Can you work these out from the model? Positions are in its coordinate system, mm. A direction names the side the tool comes from. Round coordinates to 2 decimals unless told otherwise and drop trailing zeros. Loops run counter-clockwise (first coordinate to the right, second up) from the corner with the lowest first, then second, coordinate; pieces in that order, holes last.
```python
from build123d import *

# Parameters (mm, degrees)
ESQUISSE1_W             = 30
ESQUISSE1_H             = 20
BOSS_EXTRU_1_DEPTH      = 2
ESQUISSE2_R             = 4.5
BOSS_EXTRU_2_DEPTH      = 30
ESQUISSE4_R             = 6.5
BOSS_EXTRU_3_DEPTH      = 17
CONG_1_R                = 2
ESQUISSE5_W             = 3
ESQUISSE5_H             = 5.5
ENL_V_MAT_EXTRU_1_DEPTH = 3
ESQUISSE6_R             = 1.5
ENL_V_MAT_EXTRU_2_DEPTH = 47.904157662


with BuildPart() as part:
    # Esquisse1 → Boss.-Extru.1 (new body)
    with BuildSketch(Plane.XY):
        with Locations((15, 10)):
            Rectangle(ESQUISSE1_W, ESQUISSE1_H)
    extrude(amount=BOSS_EXTRU_1_DEPTH)

    # Esquisse2 → Boss.-Extru.2 (add)
    with BuildSketch(Plane.XY.offset(2)):
        with Locations((12, 9.999053637)):
            Circle(ESQUISSE2_R)
    extrude(amount=BOSS_EXTRU_2_DEPTH)

    # Esquisse4 → Boss.-Extru.3 (add)
    with BuildSketch(Plane.XY.offset(2)):
        with Locations(Location((12, 10, 0), (0, 0, 180))):
            Circle(ESQUISSE4_R)
    extrude(amount=BOSS_EXTRU_3_DEPTH)

    # Cong_1
    cong_1_edges = [part.edges().sort_by_distance(p)[0] for p in [
        (18.5, 10, 2),
        (7.5, 9.999053637, 19),
    ]]
    fillet(cong_1_edges, radius=CONG_1_R)

    # Esquisse5 → Enl_v. mat.-Extru.1 (cut)
    with BuildSketch(Plane(origin=(0, 0, 0), x_dir=(-1, 0, 0), z_dir=(0, 0, -1))):
        with Locations((-3.5, 14)):
            Rectangle(ESQUISSE5_W, ESQUISSE5_H)
        with Locations((-3.5, 6.5)):
            Rectangle(ESQUISSE5_W, ESQUISSE5_H)
    extrude(amount=-ENL_V_MAT_EXTRU_1_DEPTH, mode=Mode.SUBTRACT)

    # Esquisse6 → Enl_v. mat.-Extru.2 (cut, through all)
    with BuildSketch(Plane.XY.offset(2)):
        with Locations((27, 13.5)):
            Circle(ESQUISSE6_R)
        with Locations((27, 6.5)):
            Circle(ESQUISSE6_R)
    extrude(amount=-ENL_V_MAT_EXTRU_2_DEPTH, mode=Mode.SUBTRACT)


solid = part.part
```
(1) Suppose I cut it at D-D (y = 1). Write out the boundary of the cut face in (x, z).
(2) Suppose I cut it at A-A (x = 2.5). Write out the boundary of the cut face in (y, z), then the cut area to 3 significant figures.
(3) If I drill on line 1 (Y direction, x = 27, z = 1.5); line 2 (Z direction, x = 20, y = 17.25); line 3 (Z direction, x = 5.5, y = 5.25), over which ranges is the centre line in solid material (lowest first)?
(4) We'd pull the mould along X, two halves only. Please class faces 4 (the flat face through (15, 0, 1)), 5 (the flat face through (4, 3.75, 1)), 6 (the flat face through (30, 10, 1)): released by +X, released by -X, zero draft, split by the parting line, or undercut.
(5) For pin 1 (2 mm diameter, centred on y = 14.5, z = 15, fed in from -X); pin 2 (1.5 mm diameter, centred on y = 12, z = 12.5, fed in from +X); pin 3 (4 mm diameter, centred on y = 16, z = 11, fed in from +X); pin 4 (1.8 mm diameter, centred on x = 27, y = 6.5, fed in from +Z), each with a flat end and sliding along its axis, tell me the tip position at first contact or that it passes through.
(6) Which directions (+Z, -Z, +X, -X, +Y, -Y) give clear straight access to the entire face, cutting with the end or side of a thin tool? Please do faces 1 (the flat face through (21, 10, 2)), 2 (the flat face through (15, 10, 0)), 3 (the flat face through (2, 14, 1)).
(7) Suppose I cut it at B-B (z = 25.5). Write out the boundary of the cut face in (x, y).
(8) Suppose I cut it at C-C (y = 13.5). Give the number of separate pieces and of enclosed holes in the cut face, then the cut area to 3 significant figures.
Check result:
1. outline: (0, 0) - (30, 0) - (30, 2) - (0, 2) - close
2. outline: (0, 0) - (3.75, 0) - (3.75, 2) - (0, 2) - close; (9.25, 0) - (11.25, 0) - (11.25, 2) - (9.25, 2) - close; (16.75, 0) - (20, 0) - (20, 2) - (16.75, 2) - close
2. area: 18.0 mm2
3. line 1: y = 0 to 5, 8 to 12, 15 to 20
3. line 2: z = 0 to 2
3. line 3: z = 0 to 2.05
4. face 4: zero draft
4. face 5: undercut
4. face 6: released by +X
5. pin 1: stops at x = 6.52
5. pin 2: stops at x = 18.38
5. pin 3: stops at x = 17.12
5. pin 4: passes through
6. face 1: +Z
6. face 2: -Z, +X, -X, +Y, -Y
6. face 3: +Z, -Z
7. outline: circle Ø9 at (12, 10)
8. separate pieces: 3
8. enclosed holes: 0
8. area: 312 mm2
